```python
from build123d import *

# Parameters (mm, degrees)
SKETCH1_W           = 50
SKETCH1_H           = 60
SKETCH1_R           = 1.6
SKETCH1_R_2         = 9
BOSS_EXTRUDE1_DEPTH = 3
SKETCH2_W           = 6
SKETCH2_H           = 35
BOSS_EXTRUDE2_DEPTH = 3
SKETCH3_R           = 0.8
CUT_EXTRUDE1_DEPTH  = 42.146081223


with BuildPart() as part:
    # Sketch1 → Boss-Extrude1 (new body)
    with BuildSketch(Plane.XY):
        Rectangle(SKETCH1_W, SKETCH1_H)
        with Locations((0, 12.5)):
            Circle(SKETCH1_R, mode=Mode.SUBTRACT)
        with Locations((10.825317547, 6.25)):
            Circle(SKETCH1_R, mode=Mode.SUBTRACT)
        with Locations((10.825317547, -6.25)):
            Circle(SKETCH1_R, mode=Mode.SUBTRACT)
        with Locations((0, -12.5)):
            Circle(SKETCH1_R, mode=Mode.SUBTRACT)
        with Locations((-10.825317547, -6.25)):
            Circle(SKETCH1_R, mode=Mode.SUBTRACT)
        with Locations((-10.825317547, 6.25)):
            Circle(SKETCH1_R, mode=Mode.SUBTRACT)
        Circle(SKETCH1_R_2, mode=Mode.SUBTRACT)
    extrude(amount=BOSS_EXTRUDE1_DEPTH)

    # Sketch2 → Boss-Extrude2 (add)
    with BuildSketch(Plane.XY.offset(3)):
        with Locations((-25, 0)):
            Rectangle(SKETCH2_W, SKETCH2_H)
        with Locations((25, 0)):
            Rectangle(SKETCH2_W, SKETCH2_H)
    extrude(amount=-BOSS_EXTRUDE2_DEPTH)

    # Sketch3 → Cut-Extrude1 (cut, through all)
    with BuildSketch(Plane.XY.offset(3)):
        with Locations((-25, 17.5)):
            Circle(SKETCH3_R)
        with Locations((-25, -17.5)):
            Circle(SKETCH3_R)
        with Locations((25, 17.5)):
            Circle(SKETCH3_R)
        with Locations((25, -17.5)):
            Circle(SKETCH3_R)
    extrude(amount=-CUT_EXTRUDE1_DEPTH, mode=Mode.SUBTRACT)


solid = part.part
```
Can you work these out from the model? Positions are in its coordinate system, mm. A direction names the side the tool comes from. Coordinates: 2 decimals unless noted, no trailing zeros. Write each loop counter-clockwise with the first axis right and the second up, starting at its lowest first coordinate (ties: lowest second). Pieces come first, ordered by that corner, then holes. Notation, with made-up numbers: M 5.5,2.25 L 35.5,2.25 A21 cw 35.5,24.25 Z; hole C -15.5,45 d5. An arc over 180 degrees is marked long. Answer as CSV lines item,"result".
Item 1: Imagine slicing it at B-B on z = 0.45. List the corners of the cut face in (x, y) for me, plus the area to 3 significant figures.
Geometry results:
outline,"M -28,-17.5 L -25.8,-17.5 A0.8 cw long -25,-18.3 L -25,-30 L 25,-30 L 25,-18.3 A0.8 cw long 25.8,-17.5 L 28,-17.5 L 28,17.5 L 25.8,17.5 A0.8 cw long 25,18.3 L 25,30 L -25,30 L -25,18.3 A0.8 cw long -25.8,17.5 L -28,17.5 Z; hole C -10.83,-6.25 d3.2; hole C -10.83,6.25 d3.2; hole C 0,0 d18; hole C 0,-12.5 d3.2; hole C 0,12.5 d3.2; hole C 10.83,-6.25 d3.2; hole C 10.83,6.25 d3.2"
area,"2,900 mm2"
Item 2: Imagine slicing it at A-A on y = -12.5. List the corners of the cut face in (x, z) for me, plus the area to 3 significant figures.
Geometry results:
outline,"M -28,0 L -1.6,0 L -1.6,3 L -28,3 Z; M 1.6,0 L 28,0 L 28,3 L 1.6,3 Z"
area,"158 mm2"
Item 3: Please list where these lines run through material, in increasing order: line 1 along Y through (x, z) = (0, 1.35); line 2 along Y through (x, z) = (-11, 0.55); line 3 along Y through (x, z) = (-12, 1.65).
Geometry results:
line 1,"y = -30 to -14.1, -10.9 to -9, 9 to 10.9, 14.1 to 30"
line 2,"y = -30 to -7.84, -4.66 to 4.66, 7.84 to 30"
line 3,"y = -30 to -7.34, -5.16 to 5.16, 7.34 to 30"
Item 4: Imagine slicing it at D-D on y = -6.25. List the corners of the cut face in (x, z) for me.
Geometry results:
outline,"M -28,0 L -12.43,0 L -12.43,3 L -28,3 Z; M -9.23,0 L -6.48,0 L -6.48,3 L -9.23,3 Z; M 6.48,0 L 9.23,0 L 9.23,3 L 6.48,3 Z; M 12.43,0 L 28,0 L 28,3 L 12.43,3 Z"
Item 5: We'd pull the mould along X, two halves only. Please class faces 5 (the cylindrical face through (-1.172, 8.923, 1.479)), 6 (the flat face through (25, -24, 1)), 7 (the flat face through (6, 7, 3)): +X half, -X half, draft (parallel to the pull), parting line (faces both ways), or undercut.
Geometry results:
face 5,"undercut"
face 6,"+X half"
face 7,"draft"
Item 6: I'm going to push flat-ended pins straight in: P1, Ø2.5, axis at x = 0, y = 12.5, coming from the -Z side; P2, Ø2, axis at x = -25, y = -17.5, coming from the -Z side; P3, Ø1.1, axis at x = -26.5, z = 1, coming from the -Y side. Where does each tip first touch, or does it pass through?
Geometry results:
P1,"passes through"
P2,"stops at z = 0"
P3,"stops at y = -17.5"
Item 7: On a 3-axis mill with a long thin cutter (end or side, diameter ignored), from which of +Z, -Z, +X, -X, +Y, -Y can I reach the whole of each face in a straight line? I mean faces 1 (the flat face through (-27, -17.5, 2)), 2 (the flat face through (27, 17.5, 2)), 3 (the flat face through (27, -17.5, 2)), 4 (the flat face through (-25, 24, 1)). Say none if no direction works.
Geometry results:
face 1,"+Z, -Z, -X, -Y"
face 2,"+Z, -Z, +X, +Y"
face 3,"+Z, -Z, +X, -Y"
face 4,"+Z, -Z, -X, +Y"
Item 8: Imagine slicing it at C-C on x = 0. List the corners of the cut face in (y, z) for me.
Geometry results:
outline,"M -30,0 L -14.1,0 L -14.1,3 L -30,3 Z; M -10.9,0 L -9,0 L -9,3 L -10.9,3 Z; M 9,0 L 10.9,0 L 10.9,3 L 9,3 Z; M 14.1,0 L 30,0 L 30,3 L 14.1,3 Z"
